from build123d import *

# Parameters (mm, degrees)
SKETCH1_W           = 120
SKETCH1_H           = 160
BOSS_EXTRUDE1_DEPTH = 30
SKETCH2_W           = 105
SKETCH2_H           = 145
CUT_EXTRUDE1_DEPTH  = 12
SKETCH3_R           = 4
BOSS_EXTRUDE2_DEPTH = 8


with BuildPart() as part:
    # Sketch1 → Boss-Extrude1 (new body)
    with BuildSketch(Plane(origin=(0, 0, 0), x_dir=(1, 0, 0), z_dir=(0, 1, 0))):
        Rectangle(SKETCH1_W, SKETCH1_H)
    extrude(amount=BOSS_EXTRUDE1_DEPTH)

    # Sketch2 → Cut-Extrude1 (cut)
    with BuildSketch(Plane(origin=(0, 30, 0), x_dir=(1, 0, 0), z_dir=(0, 1, 0))):
        Rectangle(SKETCH2_W, SKETCH2_H)
    extrude(amount=-CUT_EXTRUDE1_DEPTH, mode=Mode.SUBTRACT)

    # Sketch3 → Boss-Extrude2 (add)
    with BuildSketch(Plane(origin=(0, 18, 0), x_dir=(1, 0, 0), z_dir=(0, 1, 0))):
        with Locations(Location((-21.5, -21.5, 0), (0, 0, 90))):
            Circle(SKETCH3_R)
        with Locations(Location((25, 25, 0), (0, 0, 90))):
            Circle(SKETCH3_R)
        with Locations(Location((-36.7, -35.3, 0), (0, 0, 90))):
            Circle(SKETCH3_R)
        with Locations(Location((36.7, -35.3, 0), (0, 0, 90))):
            Circle(SKETCH3_R)
        with Locations(Location((36.7, -60.7, 0), (0, 0, 90))):
            Circle(SKETCH3_R)
        with Locations(Location((-36.7, -60.7, 0), (0, 0, 90))):
            Circle(SKETCH3_R)
        with Locations(Location((36.7, 33.409623616, 0), (0, 0, 90))):
            Circle(SKETCH3_R)
        with Locations(Location((-36.7, 33.409623616, 0), (0, 0, 90))):
            Circle(SKETCH3_R)
        with Locations(Location((-36.7, 52.809623616, 0), (0, 0, 90))):
            Circle(SKETCH3_R)
        with Locations(Location((36.7, 52.809623616, 0), (0, 0, 90))):
            Circle(SKETCH3_R)
    extrude(amount=BOSS_EXTRUDE2_DEPTH)


solid = part.part
Can you work these out from the model? Positions are in its coordinate system, mm. A direction names the side the tool comes from. Give positions to 0.01 mm unless a question says otherwise; leave off trailing zeros. Loops run counter-clockwise (first coordinate to the right, second up) from the corner with the lowest first, then second, coordinate; pieces in that order, holes last. Notation, with made-up numbers: M 30.5,13 L 45.5,13 A24 ccw 45.5,43 Z; hole C 73,10 d8. An arc over 180 degrees is marked long. One line per item, written item: value. Start each with the question number.
1) Thinking about a two-plate mould opening in Z: for faces 1 (the face through (60, 15, 1)), 2 (the face through (32.734, 21.944, -52.289)), which applies, +Z half, -Z half, draft (parallel to the pull), parting line (faces both ways), or undercut?
2) If we section it at B-B, the plane x = -3: Write out the boundary of the cut face in (y, z).
3) I'm going to push flat-ended pins straight in: pin 1 (4 mm diameter, centred on x = -19.5, z = 23.5, fed in from +Y); pin 2 (3 mm diameter, centred on x = 24, z = 9.5, fed in from +Y). Where does each tip first touch, or does it pass through?
4) If we section it at A-A, the plane z = 21.5: Write out the boundary of the cut face in (x, y).
5) On a 3-axis mill with a long thin cutter (end or side, diameter ignored), from which of +Z, -Z, +X, -X, +Y, -Y can I reach the whole of each face in a straight line? I mean faces 3 (the face through (37, 26, -33)), 4 (the face through (-54, 30, -6)). Say none if no direction works.
6) If we section it at D-D, the plane z = 68.5: Write out the boundary of the cut face in (x, y).
7) If we section it at C-C, the plane x = 36.7: Write out the boundary of the cut face in (y, z), and give its area (3 significant figures).
8) If I drill on line 1 (Z direction, x = -20, y = 27.25); line 2 (X direction, y = 21.25, z = 14.5); line 3 (Z direction, x = -35, y = 25), over which ranges is the centre line in solid material (lowest first)? Write a range as [from, to].
Completed:
1. face 1: draft
1. face 2: undercut
2. outline: M 0,-80 L 30,-80 L 30,-72.5 L 18,-72.5 L 18,72.5 L 30,72.5 L 30,80 L 0,80 Z
3. pin 1: stops at y = 26
3. pin 2: stops at y = 18
4. outline: M -60,0 L 60,0 L 60,30 L 52.5,30 L 52.5,18 L -17.5,18 L -17.5,26 L -25.5,26 L -25.5,18 L -52.5,18 L -52.5,30 L -60,30 Z
5. face 3: +Y
5. face 4: +Z, -Z, +X, -X, +Y
6. outline: M -60,0 L 60,0 L 60,30 L 52.5,30 L 52.5,18 L -52.5,18 L -52.5,30 L -60,30 Z
7. outline: M 0,-80 L 30,-80 L 30,-72.5 L 18,-72.5 L 18,-56.81 L 26,-56.81 L 26,-48.81 L 18,-48.81 L 18,-37.41 L 26,-37.41 L 26,-29.41 L 18,-29.41 L 18,31.3 L 26,31.3 L 26,39.3 L 18,39.3 L 18,56.7 L 26,56.7 L 26,64.7 L 18,64.7 L 18,72.5 L 30,72.5 L 30,80 L 0,80 Z
7. area: 3,320 mm^2
8. line 1: z = [-80, -72.5], [72.5, 80]
8. line 2: x = [-60, -52.5], [52.5, 60]
8. line 3: z = [-80, -72.5], [-56.43, -49.19], [-37.03, -29.79], [31.68, 38.92], [57.08, 64.32], [72.5, 80]
